```python
from build123d import *

# Parameters (mm, degrees)
SKETCH1_R           = 16.7005
BOSS_EXTRUDE1_DEPTH = 19.05
SKETCH2_R           = 3.175
CUT_EXTRUDE1_DEPTH  = 32.78175
SKETCH2_3_R         = 4.7625
SKETCH2_3_R_2       = 3.175
BOSS_EXTRUDE2_DEPTH = 6.35
FILLET1_R           = 9.525
FILLET2_R           = 3.175


with BuildPart() as part:
    # Sketch1 → Boss-Extrude1 (new body)
    with BuildSketch(Plane(origin=(0, 0, 0), x_dir=(1, 0, 0), z_dir=(0, 1, 0))):
        with BuildLine():
            Line((-21.332857842, 8.73125), (-50.8, 8.73125))
            Line((-50.8, 8.73125), (-50.8, 2.794))
            Line((-50.8, 2.794), (-25.4, 2.794))
            Line((-25.4, 2.794), (-25.4, -2.794))
            Line((-25.4, -2.794), (-50.8, -2.794))
            Line((-50.8, -2.794), (-50.8, -8.73125))
            Line((-50.8, -8.73125), (-21.332857842, -8.73125))
            ThreePointArc((-21.332857842, -8.73125), (23.0505, 0), (-21.332857842, 8.73125))
        make_face()
        Circle(SKETCH1_R, mode=Mode.SUBTRACT)
    extrude(amount=BOSS_EXTRUDE1_DEPTH)

    # Sketch2 → Cut-Extrude1 (cut, through all)
    with BuildSketch(Plane.XY.offset(8.73125)):
        with Locations((-41.275, 9.525)):
            Circle(SKETCH2_R)
    extrude(amount=-CUT_EXTRUDE1_DEPTH, mode=Mode.SUBTRACT)

    # Sketch2<3> → Boss-Extrude2 (add)
    with BuildSketch(Plane.XY.offset(8.73125)):
        with Locations((-41.275, 9.525)):
            Circle(SKETCH2_3_R)
        with Locations((-41.275, 9.525)):
            Circle(SKETCH2_3_R_2, mode=Mode.SUBTRACT)
    boss_extrude2 = extrude(amount=-BOSS_EXTRUDE2_DEPTH)

    # Mirror1: Boss-Extrude2 across plane
    add(boss_extrude2.mirror(Plane.XY))

    # Fillet1
    fillet1_edges = [part.edges().sort_by_distance(p)[0] for p in [
        (-50.8, 19.05, -5.762625),
        (-21.332857842, 9.525, -8.73125),
        (-21.332857842, 9.525, 8.73125),
        (-50.8, 19.05, 5.762625),
    ]]
    fillet(fillet1_edges, radius=FILLET1_R)

    # Fillet2
    fillet2_edges = [part.edges().sort_by_distance(p)[0] for p in [
        (-50.8, 0, 5.762625),
        (-50.8, 0, -5.762625),
    ]]
    fillet(fillet2_edges, radius=FILLET2_R)


solid = part.part
```
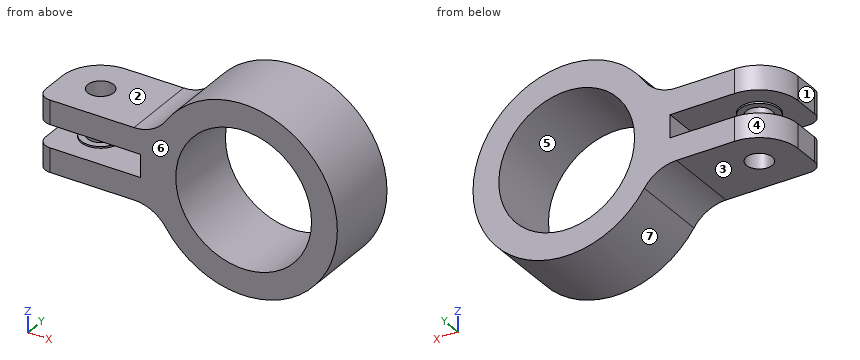
Model file for the job. Use its own axes, mm. Face numbers are marked on the shaded views. A direction names the side the tool comes from. Give positions to 0.01 mm unless a question says otherwise; leave off trailing zeros. Write each loop counter-clockwise with the first axis right and the second up, starting at its lowest first coordinate (ties: lowest second). Pieces come first, ordered by that corner, then holes. Notation, with made-up numbers: M -4,34.25 L 42,34.25 A15 cw 42,61.25 Z; hole C -30,5.5 d5. An arc over 180 degrees is marked long. Use a Markdown table: item, result.
1) Cut at D-D (z = -5). List the corners of the cut face in (x, y) (3 decimals), and give its area (3 significant figures).
Responses:
| item | result |
|---|---|
| outline | M -50.8,3.175 A3.175 ccw -47.625,0 L -15.934,0 L -15.934,19.05 L -41.275,19.05 A9.525 ccw -50.8,9.525 Z; M 15.934,0 L 22.502,0 L 22.502,19.05 L 15.934,19.05 Z; hole C -41.275,9.525 d6.35 |
| area | 736 mm2 |
2) Cut at B-B (x = 0). List the corners of the cut face in (y, z), and give its area (3 significant figures).
Responses:
| item | result |
|---|---|
| outline | M 0,-23.05 L 19.05,-23.05 L 19.05,-16.7 L 0,-16.7 Z; M 0,16.7 L 19.05,16.7 L 19.05,23.05 L 0,23.05 Z |
| area | 242 mm2 |
3) Pull direction X, two halves, no side cores. Call the marked faces 4, 5, 6 and 7: +X half, -X half, draft (parallel to the pull), parting line (faces both ways), or undercut.
Responses:
| item | result |
|---|---|
| face 4 | -X half |
| face 5 | undercut |
| face 6 | draft |
| face 7 | parting line |
4) Tool access for the marked faces 1, 2 and 3: list every direction of +Z, -Z, +X, -X, +Y, -Y with a clear straight run to the whole face (end or side of a thin tool).
Responses:
| item | result |
|---|---|
| face 1 | +Z, -Z, -X, +Y, -Y |
| face 2 | +Z, -X, +Y, -Y |
| face 3 | -Z, -X, +Y, -Y |
5) Cut at C-C (y = 7.25). Give the number of separate pieces and of enclosed holes in the cut face, and give its area (3 significant figures).
Responses:
| item | result |
|---|---|
| separate pieces | 3 |
| enclosed holes | 1 |
| area | 1,110 mm2 |
6) Pin check, flat tips, straight feed: pin 1 (6 mm diameter, centred on x = -41, y = 14, fed in from +Z); pin 2 (7.5 mm diameter, centred on x = -41.275, y = 9.525, fed in from -Z); pin 3 (2 mm diameter, centred on y = 12.5, z = 8, fed in from -X). Stop position of each tip, or through.
Responses:
| item | result |
|---|---|
| pin 1 | stops at z = 8.73 |
| pin 2 | stops at z = -8.73 |
| pin 3 | stops at x = -50.59 |
7) Cut at A-A (z = 0). List the corners of the cut face in (x, y), and give its area (3 significant figures).
Responses:
| item | result |
|---|---|
| outline | M -25.4,0 L -16.7,0 L -16.7,19.05 L -25.4,19.05 Z; M 16.7,0 L 23.05,0 L 23.05,19.05 L 16.7,19.05 Z |
| area | 287 mm2 |
8) Drill centre lines: line 1 (Z direction, x = -43.5, y = 17.75); line 2 (Z direction, x = 0, y = 5); line 3 (X direction, y = 8, z = -6.5). Where is each one in solid material? Low to high. Write a range as from..to.
Responses:
| item | result |
|---|---|
| line 1 | z = -8.73..-2.79, 2.79..8.73 |
| line 2 | z = -23.05..-16.7, 16.7..23.05 |
| line 3 | x = -50.8..-44.06, -38.49..-15.38, 15.38..22.12 |
